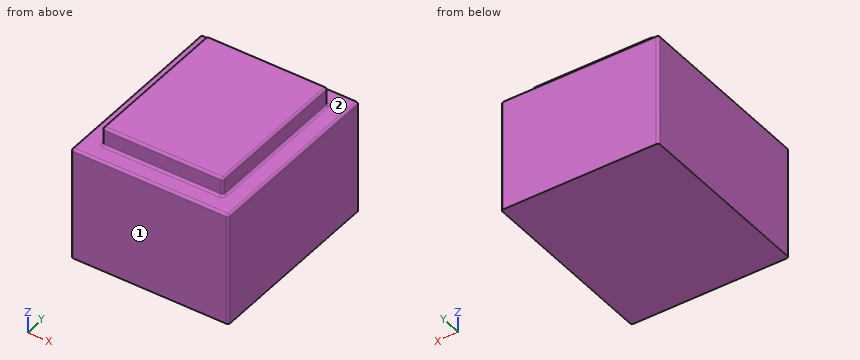
from build123d import *

# Parameters (mm, degrees)
SKETCH_W     = 34.2
SKETCH_H     = 40.6
PAD_DEPTH    = 24.5
SKETCH001_W  = 26.2
SKETCH001_H  = 32.6
PAD001_DEPTH = 4
FILLET_R     = 0.5


with BuildPart() as part:
    # Sketch → Pad (new body)
    with BuildSketch(Plane.XY):
        Rectangle(SKETCH_W, SKETCH_H)
    extrude(amount=PAD_DEPTH)

    # Sketch001 (on Face6 of Pad) → Pad001 (join)
    with BuildSketch(Plane.XY.offset(24.5)):
        Rectangle(SKETCH001_W, SKETCH001_H)
    extrude(amount=PAD001_DEPTH)

    # Fillet
    fillet_edges = [part.edges().sort_by_distance(p)[0] for p in [
        (0, -16.3, 28.5),
        (-13.1, 0, 28.5),
        (13.1, 0, 28.5),
        (0, 16.3, 28.5),
        (0, 20.3, 24.5),
        (17.1, 0, 24.5),
        (0, -20.3, 24.5),
        (-17.1, 0, 24.5),
        (-13.1, -16.3, 26.5),
        (0, -16.3, 24.5),
        (13.1, -16.3, 26.5),
        (13.1, 0, 24.5),
        (13.1, 16.3, 26.5),
        (0, 16.3, 24.5),
        (-13.1, 16.3, 26.5),
        (-13.1, 0, 24.5),
        (-17.1, 20.3, 12.25),
        (17.1, -20.3, 12.25),
        (17.1, 20.3, 12.25),
        (-17.1, -20.3, 12.25),
    ]]
    fillet(fillet_edges, radius=FILLET_R)


solid = part.part
The listing builds one solid part. Answer for the finished solid, in the listing's coordinates (mm). Face numbers are marked on the shaded views. A direction names the side the tool comes from. Give positions to 0.01 mm unless a question says otherwise; leave off trailing zeros. Loops run counter-clockwise (first coordinate to the right, second up) from the corner with the lowest first, then second, coordinate; pieces in that order, holes last.
Item 1: Each of these flat-tipped pins is pushed along its axis until it touches: pin 1 Ø0.9 at (y, z) = (0, 27) entering from +X; pin 2 Ø2.5 at (y, z) = (5, 26.5) entering from -X; pin 3 Ø1.5 at (x, z) = (0, 26.5) entering from +Y. Where does it stop, or does it pass through?
Derived:
pin 1: stops at x = 13.1
pin 2: stops at x = -13.1
pin 3: stops at y = 16.3
Item 2: A tool of negligible diameter and unlimited length cuts with its end or side. For the marked faces 1 and 2, from which of +Z, -Z, +X, -X, +Y, -Y can it reach the whole face along a straight path? Write none if from no direction.
Derived:
face 1: +Z, -Z, +X, -X, -Y
face 2: +Z
Item 3: A cutting plane is placed at A-A (x = 2.5). Give the vertices of the cut face in (y, z), then the cut area to 3 significant figures.
Derived:
outline: (-20.3, 0) - (20.3, 0) - (20.3, 24) arc R0.5 ccw to (19.8, 24.5) - (16.8, 24.5) arc R0.5 cw to (16.3, 25) - (16.3, 28) arc R0.5 ccw to (15.8, 28.5) - (-15.8, 28.5) arc R0.5 ccw to (-16.3, 28) - (-16.3, 25) arc R0.5 cw to (-16.8, 24.5) - (-19.8, 24.5) arc R0.5 ccw to (-20.3, 24) - close
area: 1,120 mm2
Item 4: Find the intervals of material crossed by line 1 along Y through (x, z) = (9.5, 25.75); line 2 along Z through (x, y) = (-11, 18.5); line 3 along X through (y, z) = (10.5, 26.25), in increasing order.
Derived:
line 1: y = -16.3 to 16.3
line 2: z = 0 to 24.5
line 3: x = -13.1 to 13.1
Item 5: A cutting plane is placed at B-B (y = 5). Give the vertices of the cut face in (x, z), then the cut area to 3 significant figures.
Derived:
outline: (-17.1, 0) - (17.1, 0) - (17.1, 24) arc R0.5 ccw to (16.6, 24.5) - (13.6, 24.5) arc R0.5 cw to (13.1, 25) - (13.1, 28) arc R0.5 ccw to (12.6, 28.5) - (-12.6, 28.5) arc R0.5 ccw to (-13.1, 28) - (-13.1, 25) arc R0.5 cw to (-13.6, 24.5) - (-16.6, 24.5) arc R0.5 ccw to (-17.1, 24) - close
area: 943 mm2
